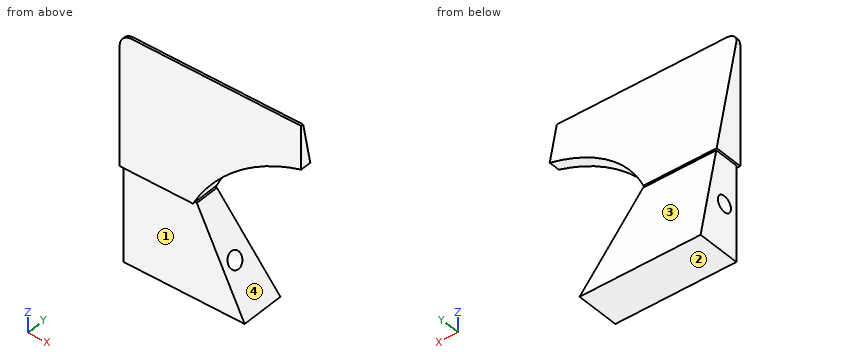
from build123d import *

# Parameters (mm, degrees)
ESBO_O1_W                                      = 130
ESBO_O1_H                                      = 20
RESSALTO_EXTRUS_O1_DEPTH                       = 95
CORTE_EXTRUS_O2_REACH                          = 22
CORTE_EXTRUS_O4_DEPTH                          = 1
CORTE_EXTRUS_O4_DEPTH_BACK                     = 131
BROCA_DE_ROSQUEAR_DE_CANO_PARA_TARRAXA_D_D     = 6.579997
BROCA_DE_ROSQUEAR_DE_CANO_PARA_TARRAXA_D_DEPTH = 10
BROCA_DE_ROSQUEAR_DE_CANO_PARA_TARRAXA_D_TIP   = 1.976830535
BROCA_DE_ROSQUEAR_DE_CANO_PARA_TARRA_2_D       = 6.579997
BROCA_DE_ROSQUEAR_DE_CANO_PARA_TARRA_2_DEPTH   = 10
BROCA_DE_ROSQUEAR_DE_CANO_PARA_TARRA_2_TIP     = 1.976830535
FILETE2_R                                      = 5
CORTE_EXTRUS_O7_DEPTH                          = 131
RESSALTO_EXTRUS_O2_REACH                       = 57.5
ESBO_O37_W                                     = 28.258303284
ESBO_O37_H                                     = 7.9
CORTE_EXTRUS_O8_REACH                          = 21.612
ESBO_O38_W                                     = 55
ESBO_O38_H                                     = 21.847631836
ESBO_O39_W                                     = 50
ESBO_O39_H                                     = 2
CORTE_EXTRUS_O9_DEPTH                          = 40.5


with BuildPart() as part:
    # Esboço1 → Ressalto-extrusão1 (new body)
    with BuildSketch(Plane.XY):
        Rectangle(ESBO_O1_W, ESBO_O1_H)
    extrude(amount=RESSALTO_EXTRUS_O1_DEPTH)

    # Esboço2 → Corte-extrusão2 (cut, up to next)
    with BuildSketch(Plane(origin=(0, 10, 0), x_dir=(1, 0, 0), z_dir=(0, 1, 0)), mode=Mode.PRIVATE) as corte_extrus_o2_sk1:
        with BuildLine():
            Line((65, 0), (-15, 0))
            Line((-15, 0), (-35, -40))
            ThreePointArc((-35, -40), (-7.92883262, -69.207295879), (30.404335441, -80))
            Line((30.404335441, -80), (65, -80))
            Line((65, -80), (65, 0))
        make_face()
    corte_extrus_o2_tool1 = extrude(corte_extrus_o2_sk1.sketch, amount=-CORTE_EXTRUS_O2_REACH, mode=Mode.PRIVATE) & part.part
    add(corte_extrus_o2_tool1.solids().sort_by_distance((21.312978, 10, 38.404428))[0], mode=Mode.SUBTRACT)

    # Esboço13 → Corte-extrusão4 (cut, two sides)
    with BuildSketch(Plane.ZY.offset(65)) as corte_extrus_o4_sk:
        Polygon((-200.200134404, 50.040026881), (0, 10), (95, -9), (295.200134404, -49.040026881), (375.280188165, 351.360241926), (-120.120080642, 450.440295688), align=None)
    extrude(amount=CORTE_EXTRUS_O4_DEPTH, mode=Mode.SUBTRACT)
    extrude(corte_extrus_o4_sk.sketch, amount=-CORTE_EXTRUS_O4_DEPTH_BACK, mode=Mode.SUBTRACT)

    # Broca de rosquear de cano para tarraxa d
    with Locations(Plane.ZY.offset(65)):
        with Locations((20, -2)):
            Hole(BROCA_DE_ROSQUEAR_DE_CANO_PARA_TARRAXA_D_D / 2, depth=BROCA_DE_ROSQUEAR_DE_CANO_PARA_TARRAXA_D_DEPTH)
            with Locations((0, 0, -(BROCA_DE_ROSQUEAR_DE_CANO_PARA_TARRAXA_D_DEPTH + BROCA_DE_ROSQUEAR_DE_CANO_PARA_TARRAXA_D_TIP / 2))):  # 118° drill point
                Cone(0, BROCA_DE_ROSQUEAR_DE_CANO_PARA_TARRAXA_D_D / 2, BROCA_DE_ROSQUEAR_DE_CANO_PARA_TARRAXA_D_TIP, mode=Mode.SUBTRACT)

    # Broca de rosquear de cano para tarra 2
    with Locations(Plane(origin=(-12, 0, -6), x_dir=(0.447213595, 0, -0.894427191), z_dir=(0.894427191, 0, 0.447213595))):
        with Locations((-26.708203932, -2)):
            Hole(BROCA_DE_ROSQUEAR_DE_CANO_PARA_TARRA_2_D / 2, depth=BROCA_DE_ROSQUEAR_DE_CANO_PARA_TARRA_2_DEPTH)
            with Locations((0, 0, -(BROCA_DE_ROSQUEAR_DE_CANO_PARA_TARRA_2_DEPTH + BROCA_DE_ROSQUEAR_DE_CANO_PARA_TARRA_2_TIP / 2))):  # 118° drill point
                Cone(0, BROCA_DE_ROSQUEAR_DE_CANO_PARA_TARRA_2_D / 2, BROCA_DE_ROSQUEAR_DE_CANO_PARA_TARRA_2_TIP, mode=Mode.SUBTRACT)

    # Filete2
    filete2_edges = [part.edges().sort_by_distance(p)[0] for p in [
        (-65, -9.5, 95),
    ]]
    fillet(filete2_edges, radius=FILETE2_R)

    # Esboço34 → Corte-extrusão7 (cut, through all)
    with BuildSketch(Plane.ZY.offset(65)):
        Polygon((40, -10), (40, 2), (39.5, 2.1), (39.5, -10), align=None)
        Polygon((40.5, 1.9), (40, 2), (40, -10), (40.5, -10), align=None)
    extrude(amount=-CORTE_EXTRUS_O7_DEPTH, mode=Mode.SUBTRACT)

    # Esboço37 → Ressalto-extrusão2 (add, up to next)
    with BuildSketch(Plane.XY.offset(39.5), mode=Mode.PRIVATE) as ressalto_extrus_o2_sk1:
        with Locations((-49.870848358, -3.05)):
            Rectangle(ESBO_O37_W, ESBO_O37_H)
    ressalto_extrus_o2_tool1 = extrude(ressalto_extrus_o2_sk1.sketch, amount=RESSALTO_EXTRUS_O2_REACH, mode=Mode.PRIVATE) - part.part
    add(ressalto_extrus_o2_tool1.solids().sort_by_distance((-49.870848, -3.05, 39.5))[0])

    # Esboço38 → Corte-extrusão8 (cut, up to next)
    with BuildSketch(Plane(origin=(0, 9.615384615, 1.923076923), x_dir=(1, 0, 0), z_dir=(0, 0.980580676, 0.196116135)), mode=Mode.PRIVATE) as corte_extrus_o8_sk1:
        with Locations((37.5, -84.932685446)):
            Rectangle(ESBO_O38_W, ESBO_O38_H)
    corte_extrus_o8_tool1 = extrude(corte_extrus_o8_sk1.sketch, amount=-CORTE_EXTRUS_O8_REACH, mode=Mode.PRIVATE) & part.part
    add(corte_extrus_o8_tool1.solids().sort_by_distance((37.5, -7.041285, 85.206427))[0], mode=Mode.SUBTRACT)

    # Esboço39 → Corte-extrusão9 (cut)
    with BuildSketch(Plane(origin=(0, 0, 0), x_dir=(-1, 0, 0), z_dir=(0, 0, -1))):
        with Locations((40, -9)):
            Rectangle(ESBO_O39_W, ESBO_O39_H)
    extrude(amount=-CORTE_EXTRUS_O9_DEPTH, mode=Mode.SUBTRACT)


solid = part.part
Verification items for the finished model (mm, model axes). Face numbers are marked on the shaded views. Round coordinates to 2 decimals unless told otherwise and drop trailing zeros. Loops run counter-clockwise (first coordinate to the right, second up) from the corner with the lowest first, then second, coordinate; pieces in that order, holes last. Notation, with made-up numbers: (86, 37.5) - (124, 37.5) arc R33 ccw to (124, 70.5) - close; hole circle Ø10 at (-4, -15). An arc over 180 degrees is marked (long way). Answer in a Markdown table with one row per item. Add a question column.
Q1. Section check C-C on x = -40. Enter the section's corners in (y, z).
Q2. Section check B-B on y = 8. Enter the section's corners in (x, z), plus the area to 3 significant figures.
Q3. Gauge pin test, flat ends, axial feed: pin 1 (0.5 mm diameter, centred on y = -4.5, z = 40, fed in from -X); pin 2 (0.8 mm diameter, centred on x = -53, z = 40, fed in from -Y); pin 3 (0.8 mm diameter, centred on y = -2.5, z = 40, fed in from +X). Record the tip position at first contact, or that the pin passes through.
Q4. Material ranges on line 1 (Y direction, x = -59.5, z = 20); line 2 (Z direction, x = -28.5, y = 0.5); line 3 (Y direction, x = -5, z = 78.5), recorded low to high.
Q5. Release check for a two-part mould opening along Z. For the marked faces 1, 2, 3 and 4 record: pulls with the +Z half, pulls with the -Z half, needs draft (parallel to the pull), parting line crosses it, or undercut.
Q6. Section check D-D on z = 86.5. Enter the section's corners in (x, y).
Q7. Section check A-A on x = -57.5. Enter the section's corners in (y, z).
Found:
| question | item | result |
|---|---|---|
| 1 | outline | (-10, 40.5) - (-7, 40.5) - (-7, 39.5) - (-8, 39.5) - (-8, 0) - (10, 0) - (2.1, 39.5) - (0.9, 39.5) - (0.9, 40.5) - (1.9, 40.5) - (-9, 95) - (-10, 95) - close |
| 2 | outline | (-65, 0) - (-15, 0) - (-20, 10) - (-65, 10) - close |
| 2 | area | 475 mm² |
| 3 | pin 1 | stops at x = -64 |
| 3 | pin 2 | stops at y = -7 |
| 3 | pin 3 | stops at x = -35.74 |
| 4 | line 1 | y = -8 to -5.29, 1.29 to 6 |
| 4 | line 2 | z = 0 to 13.22, 18 to 27 |
| 4 | line 3 | y = -10 to -5.7 |
| 5 | face 1 | needs draft |
| 5 | face 2 | pulls with the -Z half |
| 5 | face 3 | pulls with the +Z half |
| 5 | face 4 | undercut |
| 6 | outline | (-65, -10) - (10, -10) - (10, -7.3) - (-65, -7.3) - close |
| 7 | outline | (-10, 40.5) - (-7, 40.5) - (-7, 39.5) - (-8, 39.5) - (-8, 0) - (10, 0) - (2.1, 39.5) - (0.9, 39.5) - (0.9, 40.5) - (1.9, 40.5) - (-9, 95) - (-10, 95) - close; hole circle Ø6.58 at (-2, 20) |
